Verification items for this drawing (mm, ordinates from the low corner). A direction names the side the tool comes from. Coordinates: 2 decimals unless noted, no trailing zeros. Write each loop counter-clockwise with the first axis right and the second up, starting at its lowest first coordinate (ties: lowest second). Pieces come first, ordered by that corner, then holes. Notation, with made-up numbers: (73, -7) -> (94, -7) arc R21 ccw to (94, 12) -> close; hole circle Ø5 at (52, 62.5). An arc over 180 degrees is marked (long way). One line per item, written item: value. Start each with the question number.
1) Sectioned sample at C-C on y = 3. Enter the section's corners in (x, z), plus the area to 3 significant figures.
2) Sectioned sample at A-A on z = 28. Enter the section's corners in (x, y).
3) Sectioned sample at B-B on x = 3.5. Enter the section's corners in (y, z).
4) Draft check along Z on the marked faces 4, 5, 6 and 7. Enter one of: +Z half, -Z half, draft (parallel to the pull), parting line (faces both ways), or undercut.
5) Gauge pin test, flat end, axial feed: P1, Ø10, axis at x = 17.5, z = 22, coming from the -Y side. Record the tip position at first contact, or that the pin passes through.
6) Sectioned sample at D-D on x = 10. Give the number of separate pieces and of enclosed holes in the cut face, plus the area to 3 significant figures.
7) Set-up check for the marked faces 1, 2 and 3: record each of +Z, -Z, +X, -X, +Y, -Y from which the full face is reachable in a straight line by a thin tool's end or side.
8) Scan lines: line 1 along Z through (x, y) = (1.25, 10); line 2 along Z through (x, y) = (7.5, 15.25); line 3 along Y through (x, z) = (17, 35). Record each from-to range of solid material in increasing order. Write a range as [from, to].
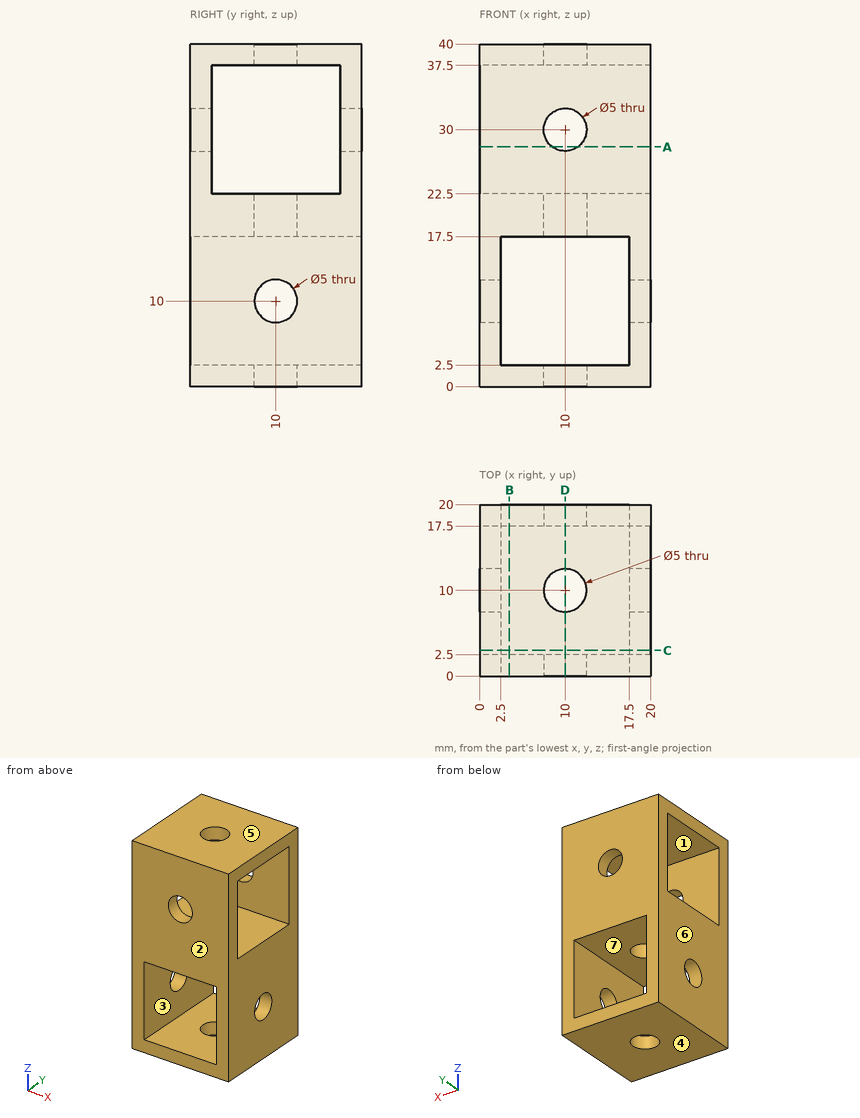
Answers:
1. outline: (0, 0) -> (20, 0) -> (20, 22.5) -> (0, 22.5) -> close; (0, 37.5) -> (20, 37.5) -> (20, 40) -> (0, 40) -> close; hole (2.5, 2.5) -> (17.5, 2.5) -> (17.5, 17.5) -> (2.5, 17.5) -> close
1. area: 275 mm2
2. outline: (0, 0) -> (8.5, 0) -> (8.5, 2.5) -> (0, 2.5) -> close; (0, 17.5) -> (8.5, 17.5) -> (8.5, 20) -> (0, 20) -> close; (11.5, 0) -> (20, 0) -> (20, 2.5) -> (11.5, 2.5) -> close; (11.5, 17.5) -> (20, 17.5) -> (20, 20) -> (11.5, 20) -> close
3. outline: (0, 0) -> (20, 0) -> (20, 2.5) -> (0, 2.5) -> close; (0, 17.5) -> (20, 17.5) -> (20, 40) -> (0, 40) -> close; hole (2.5, 22.5) -> (17.5, 22.5) -> (17.5, 37.5) -> (2.5, 37.5) -> close
4. face 4: -Z half
4. face 5: +Z half
4. face 6: draft
4. face 7: undercut
5. P1: stops at y = 0
6. separate pieces: 6
6. enclosed holes: 0
6. area: 200 mm2
7. face 1: +X, -X
7. face 2: +Z, -Z, +X, -X, -Y
7. face 3: +Y, -Y
8. line 1: z = [0, 7.5], [12.5, 22.5], [37.5, 40]
8. line 2: z = [0, 2.5], [17.5, 22.5], [37.5, 40]
8. line 3: y = [0, 2.5], [17.5, 20]
